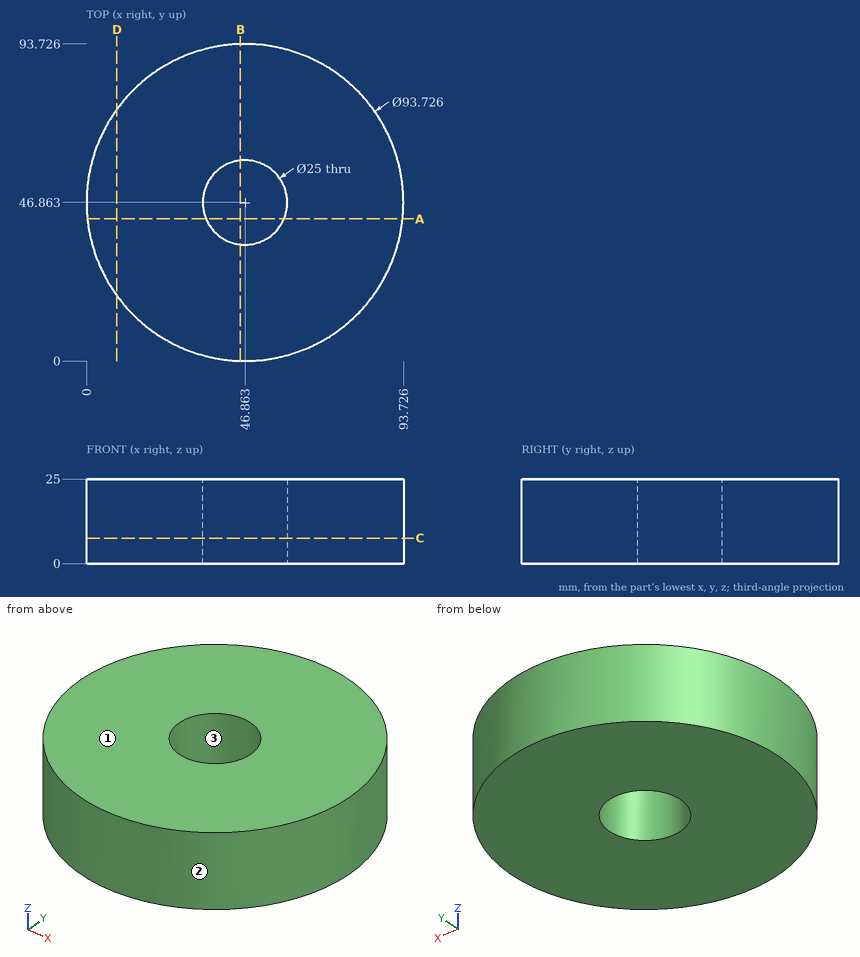
The figure shows three views and two pictorial views of one solid part (mm, origin at its lowest corner). Answer the questions. Give positions to 0.01 mm unless a question says otherwise; leave off trailing zeros. Order: outer loops, then holes, each group sorted by start corner. A loop starts at its lowest first (then second) coordinate and runs counter-clockwise, first axis right, second up. Notation, with made-up numbers: (7, 73.25) -> (39, 73.25) arc R15 cw to (39, 79.25) -> close; hole circle Ø3 at (41, 76). An arc over 180 degrees is marked (long way). Answer as CSV lines item,"result". Start each with the question number.
Q1. A cutting plane is placed at B-B (x = 45.5). Determine the outline of the cut face in (y, z) (1 decimal).
Q2. Find the intervals of material crossed by L1, parallel to Y at x = 53.5, z = 13.75 (1 decimal); L2, parallel to Y at x = 51, z = 2.5; L3, parallel to X at y = 83.5, z = 15.25 (1 decimal), in increasing order.
Q3. A cutting plane is placed at C-C (z = 7.5). Determine the outline of the cut face in (x, y) (1 decimal).
Q4. A cutting plane is placed at D-D (x = 9). Determine the outline of the cut face in (y, z).
Q5. Given pin 1 (10 mm diameter, centred on y = 54.5, z = 16.5, fed in from +X); pin 2 (12 mm diameter, centred on y = 71, z = 17, fed in from +X); pin 3 (12 mm diameter, centred on x = 18, z = 16, fed in from +Y), each flat-ended and moving along its own axis, determine where each tip first touches the part or whether it passes through.
Q6. A cutting plane is placed at A-A (y = 42). Determine the outline of the cut face in (x, z).
Q7. Determine the mould class of the marked faces 1, 2 and 3 for opening direction Y: pulls with the +Y half, pulls with the -Y half, needs draft (parallel to the pull), parting line crosses it, or undercut.
Results found:
1,outline,"(0, 0) -> (34.4, 0) -> (34.4, 25) -> (0, 25) -> close; (59.3, 0) -> (93.7, 0) -> (93.7, 25) -> (59.3, 25) -> close"
2,L1,"0.5 to 36.3, 57.5 to 93.3"
2,L2,"0.18 to 35.07, 58.66 to 93.54"
2,L3,"17.6 to 76.1"
3,outline,"circle Ø93.7 at (46.9, 46.9); hole circle Ø25 at (46.9, 46.9)"
4,outline,"(19.25, 0) -> (74.48, 0) -> (74.48, 25) -> (19.25, 25) -> close"
5,pin 1,"x = 93.65"
5,pin 2,"x = 90.07"
5,pin 3,"y = 87.77"
6,outline,"(0.25, 0) -> (35.35, 0) -> (35.35, 25) -> (0.25, 25) -> close; (58.38, 0) -> (93.47, 0) -> (93.47, 25) -> (58.38, 25) -> close"
7,face 1,"needs draft"
7,face 2,"parting line crosses it"
7,face 3,"undercut"
